Autodesk Inventor part; units mm, degrees
ref_plane "YZ Plane" through (0, 0, 0) normal (1, 0, 0) x (0, 1, 0)
ref_plane "XZ Plane" through (0, 0, 0) normal (0, 1, 0) x (-1, 0, 0)
ref_plane "XY Plane" through (0, 0, 0) normal (0, 0, 1) x (1, 0, 0)
sketch "Sketch1" plane through (0, 0, 0) normal (0, 0, 1) x (1, 0, 0)
  line L0 (0, 70) -> (0, -70) construction
  line L1 (-154, 0) -> (154, 0) construction
  line L2 (-110, 50) -> (110, 50)
  line L3 (110, 50) -> (110, -50)
  line L4 (110, -50) -> (-110, -50)
  line L5 (-110, -50) -> (-110, 50)
  point P0 (0, 0)
  dimension "d0" = 100
  dimension "d1" = 220
  dimension "d2" = 110
extrude "Extrusion1" add sketch "Sketch1" along normal blind 12.5
sketch "Sketch2" plane through (0, 0, 12.5) normal (0, 0, 1) x (1, 0, 0)
  line L0 (110, 50) -> (-110, 50) construction
  line L1 (-110, 50) -> (-110, -50) construction
  line L2 (-110, -50) -> (110, -50) construction
  line L3 (110, -50) -> (110, 50) construction
  line L4 (-60, 25) -> (60, 25) construction
  line L5 (60, 25) -> (60, -25) construction
  line L6 (60, -25) -> (-60, -25) construction
  line L7 (-60, -25) -> (-60, 25) construction
  line L8 (0, 70) -> (0, -70) construction
  line L9 (-154, 0) -> (154, 0) construction
  point P0 (0, 0)
  dimension "d5" = 50
  dimension "d6" = 120
hole "Hole1" at (-60, 25, 12.5) at (-60, -25, 12.5) at (60, -25, 12.5) at (60, 25, 12.5) direction (0, 0, -1) diameter 3.242 end through all
sketch "Sketch3" plane through (0, 0, 12.5) normal (0, 0, 1) x (1, 0, 0)
  circle A0 centre (60, -25) radius 1.621 construction
  circle A1 centre (-60, 25) radius 1.621 construction
  circle A2 centre (-60, -25) radius 1.621 construction
  circle A3 centre (60, 25) radius 1.621 construction
  line L0 (110, 50) -> (-110, 50) construction
  line L1 (-110, 50) -> (-110, -50) construction
  line L2 (-110, -50) -> (110, -50) construction
  line L3 (110, -50) -> (110, 50) construction
  line L4 (0, 70) -> (0, -70) construction
  line L5 (-154, 0) -> (154, 0) construction
  point P0 (0, 0)
  point P1 (-100, 0)
  point P2 (100, 0)
  dimension "d14" = 100
  dimension "d39" = 100
hole "Hole2" at (-100, 0, 12.5) at (100, 0, 12.5) at (0, 0, 12.5) direction (0, 0, -1) diameter 4.917 end through all
sketch "Sketch4" plane through (0, 0, 12.5) normal (0, 0, 1) x (1, 0, 0)
  circle A0 centre (-100, 0) radius 2.4585 construction
  circle A1 centre (60, -25) radius 1.621 construction
  circle A2 centre (-60, 25) radius 1.621 construction
  circle A3 centre (-60, -25) radius 1.621 construction
  circle A4 centre (60, 25) radius 1.621 construction
  line L0 (110, 50) -> (-110, 50) construction
  line L1 (-110, 50) -> (-110, -50) construction
  line L2 (-110, -50) -> (110, -50) construction
  line L3 (110, -50) -> (110, 50) construction
  line L4 (0, 70) -> (0, -70) construction
  line L5 (-154, 0) -> (154, 0) construction
  point P0 (0, 0)
  point P1 (-50, 25)
  point P2 (0, 25)
  point P3 (50, 25)
  point P4 (-50, -25)
  point P5 (0, -25)
  point P6 (50, -25)
  dimension "d22" = 50
  dimension "d23" = 25
  dimension "d26" = 50
  dimension "d29" = 50
hole "Hole3" at (-50, 25, 12.5) at (0, 25, 12.5) at (50, 25, 12.5) at (-50, -25, 12.5) at (0, -25, 12.5) at (50, -25, 12.5) direction (0, 0, -1) diameter 6 end through all counterbore diameter 10.5 counterbore depth 7
properties part number "X95carrier-to-M605-adapter-V1"
Geometry: final body of the model. Coordinates: model frame, mm. A direction names the side the tool comes from. Give positions to 0.01 mm unless a question says otherwise; leave off trailing zeros. Loops run counter-clockwise (first coordinate to the right, second up) from the corner with the lowest first, then second, coordinate; pieces in that order, holes last. Notation, with made-up numbers: (-22.5, 54.25) - (-15.5, 54.25) arc R26 cw to (-15.5, 68.25) - close; hole circle Ø1 at (57.25, -25). An arc over 180 degrees is marked (long way). One line per question, with ' | ' between items. Start each with the question number.
(1) Contact query for flat-ended pins moving along their axis: pin 1 (3 mm diameter, centred on x = 47.5, y = 22.5, fed in from +Z); pin 2 (5 mm diameter, centred on x = 0, y = 25, fed in from -Z). Output: stop coordinate, or through.
(2) Section query D-D on x = -50. Return loops of the section in (y, z), then the cut area to 3 significant figures.
(3) Section query C-C on x = 0. Return loops of the section in (y, z), then the cut area to 3 significant figures.
(4) Reachability of faces 4 (the cylindrical face through (0, 28, 3)), 5 (the cylindrical face through (-50.231, 30.245, 8.951)) from +Z, -Z, +X, -X, +Y, -Y: full face, straight path, thin tool, end or side. Return the list, or none.
(5) Section query A-A on x = 100. Return loops of the section in (y, z), then the cut area to 3 significant figures.
(6) Section query B-B on z = 8.75. Count the separate pieces of the cut face and the enclosed holes in it, then the cut area to 3 significant figures.
(7) Pull-direction query (X, two-part tool) for faces 1 (the flat face through (2, -50, 6)), 2 (the flat face through (110, 1, 6)), 3 (the flat face through (52.3, -27.3, 5.5)); classes: released by +X, released by -X, zero draft, split by the parting line, or undercut.
(8) Ray query, line 1 (Y direction, x = 50, z = 2); line 2 (Y direction, x = 0, z = 6.25); line 3 (Y direction, x = 60, z = 7). Return the intervals inside material, ascending. Write a range as from..to.
The answers:
1) pin 1: z = 5.5 | pin 2: through
2) outline: (-50, 0) - (-28, 0) - (-28, 5.5) - (-30.25, 5.5) - (-30.25, 12.5) - (-50, 12.5) - close; (-22, 0) - (22, 0) - (22, 5.5) - (19.75, 5.5) - (19.75, 12.5) - (-19.75, 12.5) - (-19.75, 5.5) - (-22, 5.5) - close; (28, 0) - (50, 0) - (50, 12.5) - (30.25, 12.5) - (30.25, 5.5) - (28, 5.5) - close | area: 1,040 mm2
3) outline: (-50, 0) - (-28, 0) - (-28, 5.5) - (-30.25, 5.5) - (-30.25, 12.5) - (-50, 12.5) - close; (-22, 0) - (-2.46, 0) - (-2.46, 12.5) - (-19.75, 12.5) - (-19.75, 5.5) - (-22, 5.5) - close; (2.46, 0) - (22, 0) - (22, 5.5) - (19.75, 5.5) - (19.75, 12.5) - (2.46, 12.5) - close; (28, 0) - (50, 0) - (50, 12.5) - (30.25, 12.5) - (30.25, 5.5) - (28, 5.5) - close | area: 976 mm2
4) face 4: +Z, -Z | face 5: +Z
5) outline: (-50, 0) - (-2.46, 0) - (-2.46, 12.5) - (-50, 12.5) - close; (2.46, 0) - (50, 0) - (50, 12.5) - (2.46, 12.5) - close | area: 1,190 mm2
6) separate pieces: 1 | enclosed holes: 13 | area: 21,400 mm2
7) face 1: zero draft | face 2: released by +X | face 3: undercut
8) line 1: -50..-28, -22..22, 28..50 | line 2: -50..-30.25, -19.75..-2.46, 2.46..19.75, 30.25..50 | line 3: -50..-26.62, -23.38..23.38, 26.62..50
